Here's how the part is built. I have some questions about the finished solid (model axes, mm). Round coordinates to 2 decimals unless told otherwise and drop trailing zeros. Answer as CSV lines item,"result".
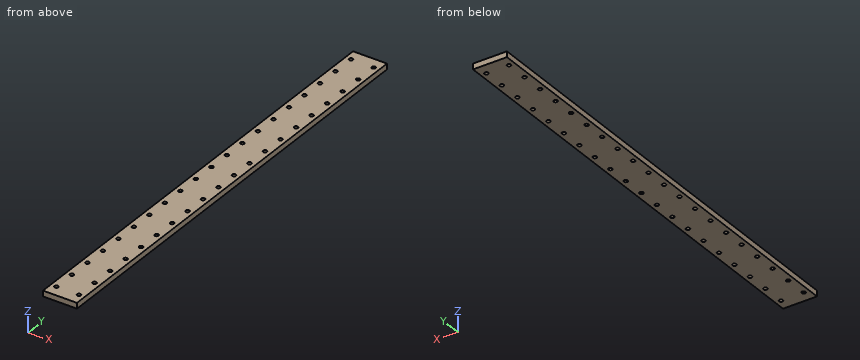
from build123d import *

# Parameters (mm, degrees)
SKETCH1_W             = 38.1
SKETCH1_H             = 508
BOSS_EXTRUDE1_DEPTH   = 3.175
F_8_CLEARANCE_HOLE1_D = 4.3053


with BuildPart() as part:
    # Sketch1 → Boss-Extrude1 (new, symmetric)
    with BuildSketch(Plane.XY):
        Rectangle(SKETCH1_W, SKETCH1_H)
    extrude(amount=BOSS_EXTRUDE1_DEPTH, both=True)

    # #8 Clearance Hole1 (through all)
    with Locations(Plane.XY.offset(3.175)):
        with Locations((-12.7, -241.3), (12.7, -241.3), (-12.7, -215.9), (12.7, -215.9), (-12.7, -190.5), (12.7, -190.5), (-12.7, -165.1), (12.7, -165.1), (-12.7, -139.7), (12.7, -139.7), (-12.7, -114.3), (12.7, -114.3), (-12.7, -88.9), (12.7, -88.9), (-12.7, -63.5), (12.7, -63.5), (-12.7, -38.1), (12.7, -38.1), (-12.7, -12.7), (12.7, -12.7), (-12.7, 12.7), (12.7, 12.7), (-12.7, 38.1), (12.7, 38.1), (-12.7, 63.5), (12.7, 63.5), (-12.7, 88.9), (12.7, 88.9), (-12.7, 114.3), (12.7, 114.3), (-12.7, 139.7), (12.7, 139.7), (-12.7, 165.1), (12.7, 165.1), (-12.7, 190.5), (12.7, 190.5), (-12.7, 215.9), (12.7, 215.9), (-12.7, 241.3), (12.7, 241.3)):
            Hole(F_8_CLEARANCE_HOLE1_D / 2)


solid = part.part
Item 1: I need wall thicknesses on L1, parallel to X at y = -40, z = -1.5. Which ranges of the line are inside material? Lowest first, please.
Results found:
L1,"x = -19.05 to -13.71, -11.69 to 11.69, 13.71 to 19.05"
Item 2: Will this pin go through, and if not, where does the flat tip stop? pin 1 (3.5 mm diameter, centred on x = 12.7, y = 215.9, fed in from +Z).
Results found:
pin 1,"passes through"
Item 3: Suppose I cut it at A-A, the plane z = -1.5. State how many separate pieces and enclosed holes the cut face has, then the cut area to 3 significant figures.
Results found:
separate pieces,"1"
enclosed holes,"40"
area,"18,800 mm²"
